Geometry check sheet. Reference: the model listing, model coordinates, mm. Face numbers are marked on the shaded views. A direction names the side the tool comes from. Round coordinates to 2 decimals unless told otherwise and drop trailing zeros. Order: outer loops, then holes, each group sorted by start corner. A loop starts at its lowest first (then second) coordinate and runs counter-clockwise, first axis right, second up. Notation, with made-up numbers: (64, 9) -> (103, 9) arc R38 ccw to (103, 48) -> close; hole circle Ø9 at (-8.75, 52.5). An arc over 180 degrees is marked (long way). Answer as a JSON object with one key per item and string values. Group by question number.
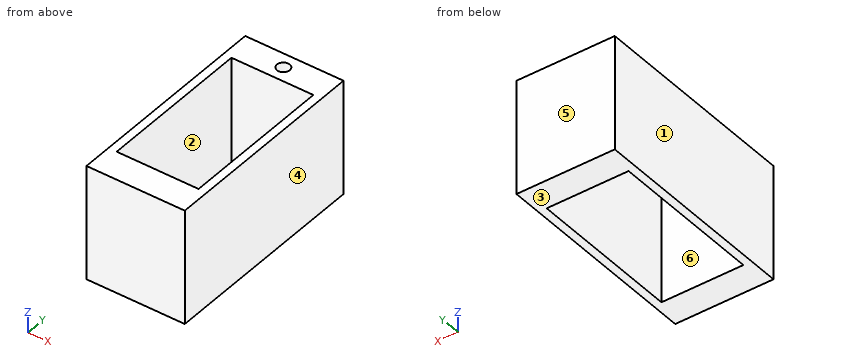
from build123d import *

# Parameters (mm, degrees)
SKETCH2_W           = 15
SKETCH2_H           = 32.5
BOSS_EXTRUDE1_DEPTH = 17.5
SKETCH3_W           = 12.5
SKETCH3_H           = 23.5
CUT_EXTRUDE1_DEPTH  = 17.5
SKETCH5_R           = 0.975
CUT_EXTRUDE2_DEPTH  = 8


with BuildPart() as part:
    # Sketch2 → Boss-Extrude1 (new body)
    with BuildSketch(Plane.XY):
        with Locations((-16.112359551, -1.991573034)):
            Rectangle(SKETCH2_W, SKETCH2_H)
    extrude(amount=BOSS_EXTRUDE1_DEPTH)

    # Sketch3 → Cut-Extrude1 (cut)
    with BuildSketch(Plane(origin=(0, 0, 0), x_dir=(-1, 0, 0), z_dir=(0, 0, -1))):
        with Locations((16.112359551, -1.991573034)):
            Rectangle(SKETCH3_W, SKETCH3_H)
    extrude(amount=-CUT_EXTRUDE1_DEPTH, mode=Mode.SUBTRACT)

    # Sketch5 → Cut-Extrude2 (cut)
    with BuildSketch(Plane.XY.offset(17.5)):
        with Locations((-16.112359551, 12.008426966)):
            Circle(SKETCH5_R)
    extrude(amount=-CUT_EXTRUDE2_DEPTH, mode=Mode.SUBTRACT)


solid = part.part
Item 1: Set-up check for the marked faces 5 and 6: record each of +Z, -Z, +X, -X, +Y, -Y from which the full face is reachable in a straight line by a thin tool's end or side.
Item 2: Sectioned sample at B-B, the plane x = -13.5. Enter the section's corners in (y, z).
Item 3: Mould release check, pull along X, two halves, no side actions. Record for the marked faces 1, 2, 3 and 4: pulls with the +X half, pulls with the -X half, needs draft (parallel to the pull), parting line crosses it, or undercut.
Item 4: Depth check by flat-ended pin: pin 1 Ø8 at (x, y) = (-16, 1) entering from +Z (3 decimals). Enter the tip coordinate at first touch or a pass-through.
Item 5: Thickness scan on L1, parallel to Y at x = -15.5, z = 4; L2, parallel to X at y = 8, z = 16.25. Record the ranges inside material, lowest first.
Item 6: Sectioned sample at D-D, the plane z = 10.5. Enter the section's corners in (x, y) (3 decimals), then the cut area to 3 significant figures.
Item 7: Sectioned sample at C-C, the plane z = 4.5. Enter the section's corners in (x, y), then the cut area to 3 significant figures.
Item 8: Sectioned sample at A-A, the plane y = 0.5. Enter the section's corners in (x, z).
Result:
{
 "1": {"face 5": "+Z, -Z, +X, -X, +Y", "face 6": "+Z, -Z"},
 "2": {"outline": "(-18.24, 0) -> (-13.74, 0) -> (-13.74, 17.5) -> (-18.24, 17.5) -> close; (9.76, 0) -> (14.26, 0) -> (14.26, 17.5) -> (9.76, 17.5) -> close"},
 "3": {"face 1": "pulls with the -X half", "face 2": "undercut", "face 3": "needs draft", "face 4": "pulls with the +X half"},
 "4": {"pin 1": "passes through"},
 "5": {"L1": "y = -18.24 to -13.74, 9.76 to 14.26", "L2": "x = -23.61 to -22.36, -9.86 to -8.61"},
 "6": {"outline": "(-23.612, -18.242) -> (-8.612, -18.242) -> (-8.612, 14.258) -> (-23.612, 14.258) -> close; hole (-22.362, -13.742) -> (-9.862, -13.742) -> (-9.862, 9.758) -> (-22.362, 9.758) -> close; hole circle Ø1.95 at (-16.112, 12.008)", "area": "191 mm2"},
 "7": {"outline": "(-23.61, -18.24) -> (-8.61, -18.24) -> (-8.61, 14.26) -> (-23.61, 14.26) -> close; hole (-22.36, -13.74) -> (-9.86, -13.74) -> (-9.86, 9.76) -> (-22.36, 9.76) -> close", "area": "194 mm2"},
 "8": {"outline": "(-23.61, 0) -> (-22.36, 0) -> (-22.36, 17.5) -> (-23.61, 17.5) -> close; (-9.86, 0) -> (-8.61, 0) -> (-8.61, 17.5) -> (-9.86, 17.5) -> close"}
}
